Read the model definition and answer for the solid it produces. Units are mm, in the model's axes. Face numbers are marked on the shaded views. A direction names the side the tool comes from. Coordinates: 2 decimals unless noted, no trailing zeros. Loops run counter-clockwise (first coordinate to the right, second up) from the corner with the lowest first, then second, coordinate; pieces in that order, holes last. Notation, with made-up numbers: (36, 41.25) - (41, 41.25) arc R32 ccw to (41, 67.25) - close; hole circle Ø1 at (77, -17). An arc over 180 degrees is marked (long way). Use one line per item in the form item = value.
from build123d import *

# Parameters (mm, degrees)
F0_W     = 120
F0_H     = 120
F1_DEPTH = 246
F2_W     = 100
F2_H     = 100
F3_DEPTH = 40
F4_W     = 85
F4_H     = 85
F5_DEPTH = 60


with BuildPart() as f1:
    # F0 (on Top) → F1 (new body)
    with BuildSketch(Plane.XY):
        with Locations((60, 60)):
            Rectangle(F0_W, F0_H)
    extrude(amount=F1_DEPTH)

    # F2 (on face) → F3 (cut)
    with BuildSketch(Plane(origin=(0, 0, 0), x_dir=(1, 0, 0), z_dir=(0, 0, -1))):
        with Locations((60, -60)):
            Rectangle(F2_W, F2_H)
    extrude(amount=-F3_DEPTH, mode=Mode.SUBTRACT)

    # F4 (on face) → F5 (cut)
    with BuildSketch(Plane.XY.offset(246)):
        with Locations((60, 60)):
            Rectangle(F4_W, F4_H)
    extrude(amount=-F5_DEPTH, mode=Mode.SUBTRACT)


solid = f1.part
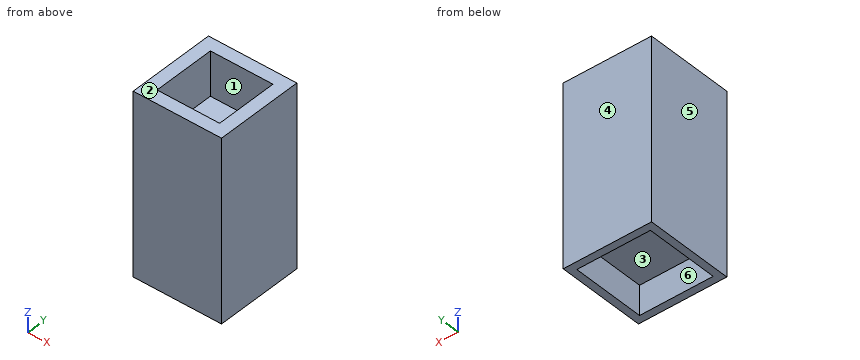
Item 1: The part is cut by section B-B on y = 15. Give the vertices of the cut face in (x, z), plus the area to 3 significant figures.
Results below:
outline = (0, 0) - (10, 0) - (10, 40) - (110, 40) - (110, 0) - (120, 0) - (120, 246) - (0, 246) - close
area = 25,500 mm²
Item 2: Each of these flat-tipped pins is pushed along its axis until it touches: P1, Ø10, axis at x = 50, y = 28.5, coming from the -Z side; P2, Ø8, axis at x = 57.5, y = 28.5, coming from the +Z side. Where does it stop, or does it pass through?
Results below:
P1 = 40
P2 = 186
Item 3: Find the intervals of material crossed by L1, parallel to Y at x = 46.5, z = 231; L2, parallel to Z at x = 48, y = 37; L3, parallel to Y at x = 109.5, z = 20, in increasing order.
Results below:
L1 = 0 to 17.5, 102.5 to 120
L2 = 40 to 186
L3 = 0 to 10, 110 to 120
Item 4: The part is cut by section C-C on x = 44. Give the vertices of the cut face in (y, z).
Results below:
outline = (0, 0) - (10, 0) - (10, 40) - (110, 40) - (110, 0) - (120, 0) - (120, 246) - (102.5, 246) - (102.5, 186) - (17.5, 186) - (17.5, 246) - (0, 246) - close
Item 5: Which of the six approach directions +Z, -Z, +X, -X, +Y, -Y give full straight-line access (tool end or side, diameter ignored) to the marked faces 1, 2 and 3?
Results below:
face_1 = +Z
face_2 = +Z, +X, -X, +Y, -Y
face_3 = -Z
Item 6: The part is cut by section A-A on z = 222. Give the vertices of the cut face in (x, y), plus the area to 4 significant figures.
Results below:
outline = (0, 0) - (120, 0) - (120, 120) - (0, 120) - close; hole (17.5, 17.5) - (102.5, 17.5) - (102.5, 102.5) - (17.5, 102.5) - close
area = 7,175 mm²
Item 7: For a pull along X with two mould halves and no side action, classify the marked faces 4, 5 and 6 as +X half, -X half, draft (parallel to the pull), parting line (faces both ways), or undercut.
Results below:
face_4 = draft
face_5 = -X half
face_6 = undercut
